The drawing under review shows one solid part. Ordinate dimensions are in mm from its lowest x, y, z. Coordinates: 2 decimals unless noted, no trailing zeros. Write each loop counter-clockwise with the first axis right and the second up, starting at its lowest first coordinate (ties: lowest second). Pieces come first, ordered by that corner, then holes. Notation, with made-up numbers: (-18.5, 8.5) - (16.5, 8.5) arc R35 cw to (16.5, 47.5) - close; hole circle Ø1 at (-8.5, -27). An arc over 180 degrees is marked (long way). Answer as CSV lines item,"result". Start each with the question number.
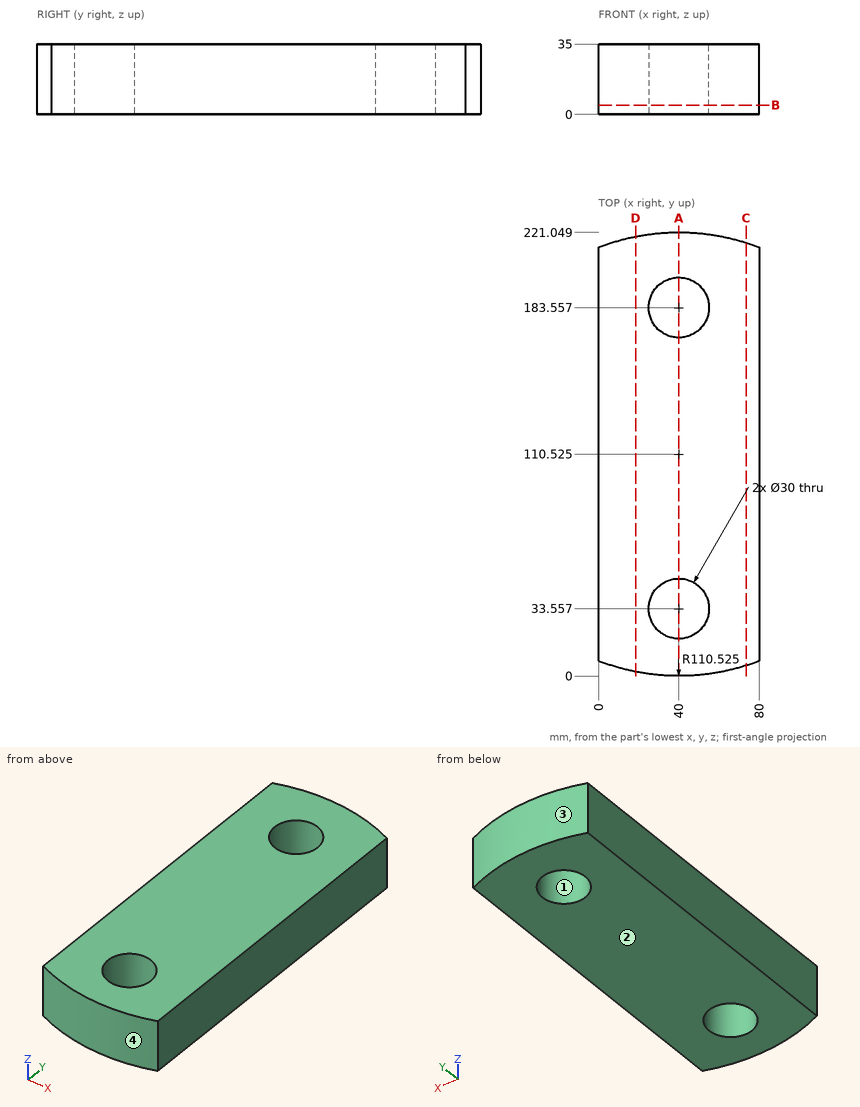
(1) For pin 1 (3 mm diameter, centred on x = 57.5, y = 22.5, fed in from -Z); pin 2 (1.5 mm diameter, centred on x = 26.5, z = 23, fed in from +Y); pin 3 (1.5 mm diameter, centred on x = 72, z = 25, fed in from +Y); pin 4 (2 mm diameter, centred on x = 13.5, z = 27.5, fed in from -Y), all flat-tipped, find the tip position at first contact; note any pin that passes through.
(2) The part is to be moulded in two halves that separate along Y. For the marked faces 1, 2, 3 and 4, say which applies: released by +Y, released by -Y, zero draft, split by the parting line, or undercut.
(3) Add section D-D on x = 18.5. Give the boundary of the cut face in (y, z), then the cut area to 3 significant figures.
(4) Wall thickness on line 1 (Y direction, x = 40, z = 17); line 2 (Y direction, x = 39, z = 10.5) (1 decimal); line 3 (X direction, y = 186, z = 5.5): over which ranges is each line inside the solid? List them lowest first.
(5) Add section C-C on x = 73.5. Give the boundary of the cut face in (y, z), then the cut area to 3 significant figures.
(6) Add section A-A on x = 40. Give the boundary of the cut face in (y, z), then the cut area to 3 significant figures.
(7) Add section B-B on z = 4.5. Give the number of separate pieces and of enclosed holes in the cut face, then the cut area to 3 significant figures.
Reported:
1,pin 1,"z = 0"
1,pin 2,"y = 220.31"
1,pin 3,"y = 216.54"
1,pin 4,"y = 2.98"
2,face 1,"undercut"
2,face 2,"zero draft"
2,face 3,"released by +Y"
2,face 4,"released by -Y"
3,outline,"(2.11, 0) - (218.94, 0) - (218.94, 35) - (2.11, 35) - close"
3,area,"7,590 mm²"
4,line 1,"0 to 18.56, 48.56 to 168.56, 198.56 to 221.05"
4,line 2,"0 to 18.6, 48.5 to 168.6, 198.5 to 221"
4,line 3,"0 to 25.2, 54.8 to 80"
5,outline,"(5.2, 0) - (215.85, 0) - (215.85, 35) - (5.2, 35) - close"
5,area,"7,370 mm²"
6,outline,"(0, 0) - (18.56, 0) - (18.56, 35) - (0, 35) - close; (48.56, 0) - (168.56, 0) - (168.56, 35) - (48.56, 35) - close; (198.56, 0) - (221.05, 0) - (221.05, 35) - (198.56, 35) - close"
6,area,"5,640 mm²"
7,separate pieces,"1"
7,enclosed holes,"2"
7,area,"15,900 mm²"
